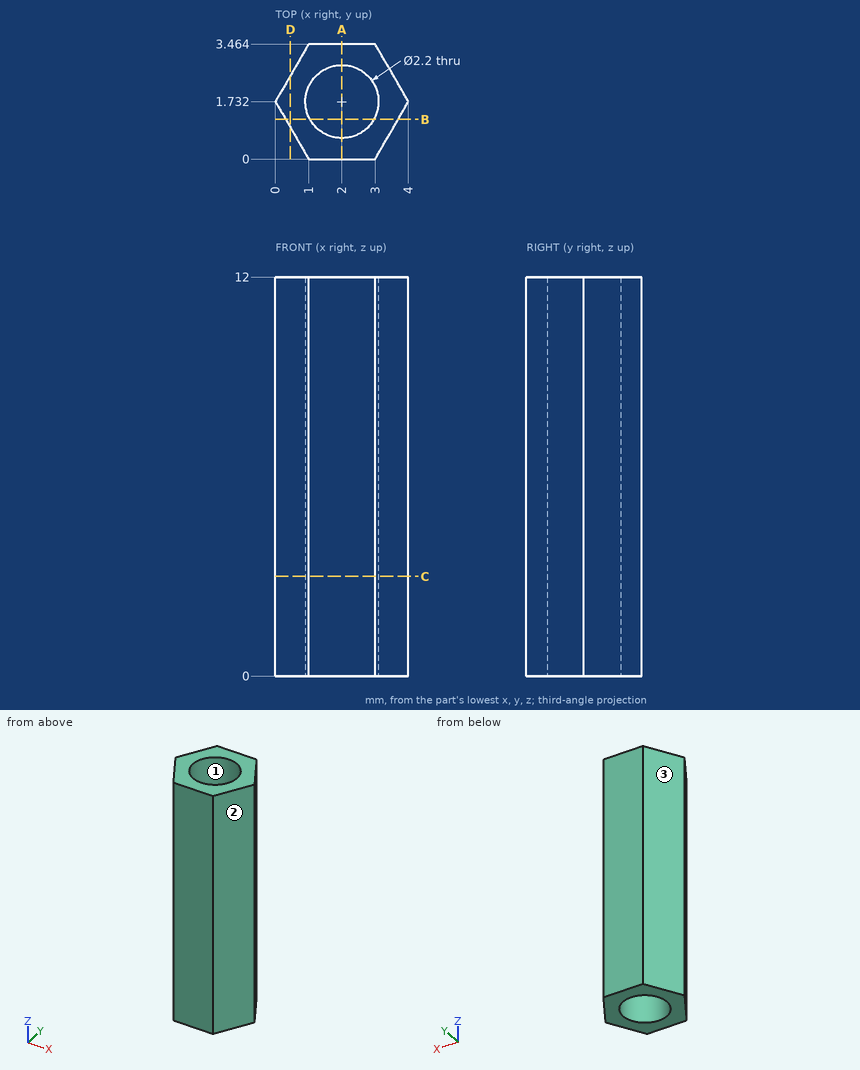
Geometry check sheet. Reference: drawing and pictorial views, mm from the part's lowest x, y, z. Give positions to 0.01 mm unless a question says otherwise; leave off trailing zeros. Order: outer loops, then holes, each group sorted by start corner. A loop starts at its lowest first (then second) coordinate and runs counter-clockwise, first axis right, second up.
1. Section check D-D, the plane x = 0.45. Enter the section's corners in (y, z), and give its area (3 significant figures).
2. Section check A-A, the plane x = 2. Enter the section's corners in (y, z).
3. Section check C-C, the plane z = 3. Enter the section's corners in (x, y), and give its area (3 significant figures).
4. Release check for a two-part mould opening along X. For the marked faces 1, 2 and 3 record: pulls with the +X half, pulls with the -X half, needs draft (parallel to the pull), parting line crosses it, or undercut.
5. Thickness scan on L1, parallel to Y at x = 2, z = 7.75; L2, parallel to X at y = 1.25, z = 10.75; L3, parallel to Y at x = 1.8, z = 1. Record the ranges inside material, lowest first.
6. Section check B-B, the plane y = 1.2. Enter the section's corners in (x, z).
Values follow:
1. outline: (0.95, 0) - (2.51, 0) - (2.51, 12) - (0.95, 12) - close
1. area: 18.7 mm2
2. outline: (0, 0) - (0.63, 0) - (0.63, 12) - (0, 12) - close; (2.83, 0) - (3.46, 0) - (3.46, 12) - (2.83, 12) - close
3. outline: (0, 1.73) - (1, 0) - (3, 0) - (4, 1.73) - (3, 3.46) - (1, 3.46) - close; hole circle Ø2.2 at (2, 1.73)
3. area: 6.59 mm2
4. face 1: undercut
4. face 2: pulls with the +X half
4. face 3: pulls with the -X half
5. L1: y = 0 to 0.63, 2.83 to 3.46
5. L2: x = 0.28 to 1.01, 2.99 to 3.72
5. L3: y = 0 to 0.65, 2.81 to 3.46
6. outline: (0.31, 0) - (1.04, 0) - (1.04, 12) - (0.31, 12) - close; (2.96, 0) - (3.69, 0) - (3.69, 12) - (2.96, 12) - close
